Geometry check sheet. Reference: the model listing, model coordinates, mm. A direction names the side the tool comes from. Coordinates: 2 decimals unless noted, no trailing zeros. Loops run counter-clockwise (first coordinate to the right, second up) from the corner with the lowest first, then second, coordinate; pieces in that order, holes last. Notation, with made-up numbers: M 75.5,77 L 102.5,77 A35 cw 102.5,115 Z; hole C 89.5,-1 d2. An arc over 180 degrees is marked long. One line per question, with ' | ' between items. Start each with the question number.
from build123d import *

# Parameters (mm, degrees)
F0_R     = 35
F1_DEPTH = 1
F2_R     = 35
F2_R_2   = 32.75
F3_DEPTH = 9
F5_DEPTH = 2
F6_W     = 10
F6_H     = 76.2
F7_DEPTH = 25.4
F8_R     = 5.08


with BuildPart() as f1:
    # F0 (on Top) → F1 (new body)
    with BuildSketch(Plane.XY):
        Circle(F0_R)
    extrude(amount=-F1_DEPTH)

    # F2 (on Top) → F3 (join)
    with BuildSketch(Plane.XY):
        Circle(F2_R)
        Circle(F2_R_2, mode=Mode.SUBTRACT)
    extrude(amount=F3_DEPTH)

    # F4 (on face) → F5 (join)
    with BuildSketch(Plane.XY.offset(9)):
        with BuildLine():
            ThreePointArc((-31.8796565226, 7.5), (-32.531686485, 3.7751654854), (-32.75, 0))
            ThreePointArc((-32.75, 0), (-32.531686485, -3.7751654854), (-31.8796565226, -7.5))
            Line((-31.8796565226, -7.5), (-30.8796565226, -7.5))
            ThreePointArc((-30.8796565226, -7.5), (-31.7774005695, 0), (-30.8796565226, 7.5))
            Line((-30.8796565226, 7.5), (-31.8796565226, 7.5))
        make_face()
        with BuildLine():
            Line((30.8796565226, -7.5), (31.8796565226, -7.5))
            ThreePointArc((31.8796565226, -7.5), (32.531686485, -3.7751654854), (32.75, 0))
            ThreePointArc((32.75, 0), (32.531686485, 3.7751654854), (31.8796565226, 7.5))
            Line((31.8796565226, 7.5), (30.8796565226, 7.5))
            ThreePointArc((30.8796565226, 7.5), (31.7774005695, 0), (30.8796565226, -7.5))
        make_face()
    extrude(amount=-F5_DEPTH)

    # F6 (on Top) → F7 (cut)
    with BuildSketch(Plane.XY):
        Rectangle(F6_W, F6_H)
    extrude(amount=F7_DEPTH, mode=Mode.SUBTRACT)

    # F8
    f8_edges = [f1.edges().sort_by_distance(p)[0] for p in [
        (-5, 33.503543, 9),
        (-5, -33.503543, 9),
        (5, -33.503543, 9),
        (5, 33.503543, 9),
    ]]
    fillet(f8_edges, radius=F8_R)


solid = f1.part
1. Thickness scan on line 1 (Z direction, x = 12, y = 8.5); line 2 (X direction, y = -27, z = 3); line 3 (Y direction, x = 14, z = 5.75). Record the ranges inside material, lowest first.
2. Sectioned sample at B-B (y = 0). Record the cut outline in (x, z).
3. Sectioned sample at C-C (x = 6). Record the cut outline in (y, z).
4. Tool access check on faces 5 (the flat face through (-32, 0, 9)), 6 (the flat face through (-5, 33, 2)), 7 (the flat face through (-32, 0, 7)), 8 (the cylindrical face through (31.777, 0.106, 8.014)). Record the directions out of +Z, -Z, +X, -X, +Y, -Y that give a thin tool (end or side, any length) a straight path to the whole face; none if there is none.
5. Draft check along X on faces 1 (the cylindrical face through (6.528, 33.263, 7.551)), 2 (the cylindrical face through (16.15, -31.05, 3.93)), 3 (the cylindrical face through (-6.528, 33.263, 7.551)), 4 (the flat face through (0, 0, -1)). Enter one of: +X half, -X half, draft (parallel to the pull), parting line (faces both ways), or undercut.
6. Sectioned sample at A-A (z = 2.5). Record the cut outline in (x, y), and give its area (3 significant figures).
7. Sectioned sample at D-D (y = -28.5). Record the cut outline in (x, z), and give its area (3 significant figures).
8. Depth check by flat-ended pin: pin 1 Ø3 at (x, z) = (12.5, 0.5) entering from +Y; pin 2 Ø1.1 at (x, z) = (-31.5, 7.5) entering from +Y; pin 3 Ø5 at (y, z) = (22, 2.5) entering from +X. Enter the tip coordinate at first touch or a pass-through.
Result:
1) line 1: z = -1 to 0 | line 2: x = -22.27 to -18.54, 18.54 to 22.27 | line 3: y = -32.08 to -29.61, 29.61 to 32.08
2) outline: M -35,-1 L 35,-1 L 35,9 L 31.78,9 L 31.78,7 L 32.75,7 L 32.75,0 L -32.75,0 L -32.75,7 L -31.78,7 L -31.78,9 L -35,9 Z
3) outline: M -34.48,-1 L 34.48,-1 L 34.48,6.95 L 32.2,6.95 L 32.2,0 L -32.2,0 L -32.2,6.95 L -34.48,6.95 Z
4) face 5: +Z, +X, -X, +Y, -Y | face 6: +Z, +Y, -Y | face 7: none | face 8: +Z
5) face 1: undercut | face 2: parting line | face 3: undercut | face 4: draft
6) outline: M -5,-34.64 L -5,-32.37 A32.75 cw -5,32.37 L -5,34.64 A35 ccw Z; M 5,-34.64 A35 ccw 5,34.64 L 5,32.37 A32.75 cw 5,-32.37 Z | area: 434 mm2
7) outline: M -20.32,-1 L 20.32,-1 L 20.32,9 L 16.13,9 L 16.13,0 L -16.13,0 L -16.13,9 L -20.32,9 Z | area: 116 mm2
8) pin 1: stops at y = 33.23 | pin 2: stops at y = 16.34 | pin 3: stops at x = 29.06
